```python
from build123d import *

# Parameters (mm, degrees)
SKETCH_1_R      = 0.3575
EXTRUDE_1_DEPTH = 1


with BuildPart() as part:
    # Эскиз1 → Бобышка-Вытянуть1 (new body)
    with BuildSketch(Plane(origin=(-34, 0, 0), x_dir=(0, -1, 0), z_dir=(-1, 0, 0))):
        with BuildLine():
            Line((-8.389166667, -1.257451802), (-8.389166667, -0.17875))
            ThreePointArc((-8.389166667, -0.17875), (-8.44152133, -0.052354663), (-8.567916667, 0))
            Line((-8.567916667, 0), (-9.470386179, 0))
            ThreePointArc((-9.470386179, 0), (-9.717011227, -0.10215544), (-9.819166667, -0.348780488))
            Line((-9.819166667, -0.348780488), (-9.819166667, -0.563811004))
            ThreePointArc((-9.819166667, -0.563811004), (-9.894763543, -0.7806486), (-10.088783486, -0.903488707))
            ThreePointArc((-10.088783486, -0.903488707), (-8.2225, -17.133890567), (-6.356216514, -0.903488707))
            ThreePointArc((-6.356216514, -0.903488707), (-6.550236457, -0.7806486), (-6.625833333, -0.563811004))
            Line((-6.625833333, -0.563811004), (-6.625833333, -0.348780488))
            ThreePointArc((-6.625833333, -0.348780488), (-6.727988773, -0.10215544), (-6.974613821, 0))
            Line((-6.974613821, 0), (-7.877083333, 0))
            ThreePointArc((-7.877083333, 0), (-8.00347867, -0.052354663), (-8.055833333, -0.17875))
            Line((-8.055833333, -0.17875), (-8.055833333, -1.257451802))
            ThreePointArc((-8.055833333, -1.257451802), (-8.006422993, -1.380832575), (-7.88550813, -1.436003154))
            ThreePointArc((-7.88550813, -1.436003154), (-8.2225, -15.728057234), (-8.55949187, -1.436003154))
            ThreePointArc((-8.55949187, -1.436003154), (-8.438577007, -1.380832575), (-8.389166667, -1.257451802))
        make_face()
        with Locations((-9.104166667, -0.741312313)):
            Circle(SKETCH_1_R, mode=Mode.SUBTRACT)
        with Locations((-7.340833333, -0.741312313)):
            Circle(SKETCH_1_R, mode=Mode.SUBTRACT)
    extrude(amount=-EXTRUDE_1_DEPTH)


solid = part.part
```
Check sheet for the modelled part. Datum: model origin and axes. Units: mm. A direction names the side the tool comes from. Round coordinates to 2 decimals unless told otherwise and drop trailing zeros. Loops run counter-clockwise (first coordinate to the right, second up) from the corner with the lowest first, then second, coordinate; pieces in that order, holes last. Notation, with made-up numbers: (-11.75, 0.5) - (-0.75, 0.5) arc R20 ccw to (-0.75, 27.5) - close; hole circle Ø1 at (-39, -27). An arc over 180 degrees is marked (long way). Write item = value, one per line. Start each with the question number.
Q1. Section check B-B (y = 2.25). Record the boundary of the cut face in (x, z).
Q2. Thickness scan on L1, parallel to Z at x = -33.8, y = 7.5; L2, parallel to Z at x = -33.2, y = 6; L3, parallel to Y at x = -33.4, z = -2.5. Record the ranges inside material, lowest first.
Q3. Access from +Z, -Z, +X, -X, +Y, -Y to the whole of each face (thin tool, end or side, straight path). Record for faces 1 (the face through (-33.5, 8.056, -0.7)), 2 (the face through (-33, 10, -16)).
Q4. Section check C-C (x = -33.8). Count the separate pieces of the cut face and the enclosed holes in it, plus the area to 3 significant figures.
Q5. Section check A-A (z = -12.25). Record the boundary of the cut face in (x, y).
Q6. Release check for a two-part mould opening along Z. For faces 3 (the face through (-33.507, 8.558, -17.127)), 4 (the face through (-33.5, 7.4, 0)), 5 (the face through (-33.51, 7.91, -15.72)) record: pulls with the +Z half, pulls with the -Z half, needs draft (parallel to the pull), parting line crosses it, or undercut.
Derived:
q1.outline = (-34, -14.56) - (-33, -14.56) - (-33, -12.51) - (-34, -12.51) - close; (-34, -4.65) - (-33, -4.65) - (-33, -3.26) - (-34, -3.26) - close
q2.L1 = -17.1 to -15.69, -1.46 to -1.06, -0.42 to 0
q2.L2 = -16.83 to -15.37, -1.78 to -0.99
q2.L3 = 3.07 to 4.46, 11.99 to 13.37
q3.face_1 = +Z, +X, -X
q3.face_2 = +Z, -Z, +X, +Y, -Y
q4.separate_pieces = 1
q4.enclosed_holes = 2
q4.area = 52.8 mm^2
q5.outline = (-34, 0.71) - (-33, 0.71) - (-33, 2.09) - (-34, 2.09) - close; (-34, 14.36) - (-33, 14.36) - (-33, 15.74) - (-34, 15.74) - close
q6.face_3 = parting line crosses it
q6.face_4 = pulls with the +Z half
q6.face_5 = undercut
